Geometry check sheet. Reference: the model listing, model coordinates, mm. A direction names the side the tool comes from. Give positions to 0.01 mm unless a question says otherwise; leave off trailing zeros. Write each loop counter-clockwise with the first axis right and the second up, starting at its lowest first coordinate (ties: lowest second). Pieces come first, ordered by that corner, then holes. Notation, with made-up numbers: M 50.25,1.25 L 106.25,1.25 A26 ccw 106.25,39.25 Z; hole C 65.25,5 d8. An arc over 180 degrees is marked long. One line per item, written item: value. Start each with the question number.
1. Cross-section at B-B on y = 54. Record the cut outline in (x, z).
2. Gauge pin test, flat ends, axial feed: pin 1 (0.8 mm diameter, centred on x = -23.5, z = 4.5, fed in from -Y); pin 2 (0.9 mm diameter, centred on y = 27, z = 19.5, fed in from -X); pin 3 (0.8 mm diameter, centred on y = 25.5, z = 3.5, fed in from +X); pin 4 (2 mm diameter, centred on x = -21.5, z = 1.5, fed in from -Y). Record the tip position at first contact, or that the pin passes through.
3. Cross-section at C-C on x = -17. Count the separate pieces of the cut face and the enclosed holes in it, then the cut area to 3 significant figures.
4. Tool access check on faces 1 (the face through (-23.5, 25, 8)), 2 (the face through (-14.949, 40.313, 16.68)), 3 (the face through (-27, 12, 3)). Record the directions out of +Z, -Z, +X, -X, +Y, -Y that give a thin tool (end or side, any length) a straight path to the whole face; none if there is none.
5. Release check for a two-part mould opening along Z. For faces 4 (the face through (0, 20, -35)), 5 (the face through (18, 37, 0)), 6 (the face through (-23.49, 27.15, 10.09)), 7 (the face through (0, 40, 20)) record: pulls with the +Z half, pulls with the -Z half, needs draft (parallel to the pull), parting line crosses it, or undercut.
6. Cross-section at A-A on y = 34. Record the cut outline in (x, z), then the cut area to 3 significant figures.
7. Scan lines: line 1 (Y direction, x = 3, z = 0); line 2 (X direction, y = 46, z = 20); line 3 (Y direction, x = 12, z = -18). Record each from-to range of solid material in increasing order.
Autodesk Inventor part; units mm, degrees
ref_plane "Work Plane1" through (0, 10, 0) normal (0, -1, 0) x (1, 0, 0)
ref_plane "Work Plane3" through (0, 0, 30) normal (1, 0, 0) x (0, 0, -1)
ref_plane "Work Plane4" through (-24, 20.5, 15) normal (0, -1, 0) x (1, 0, 0)
sketch "Sketch1" plane through (0, 0, 0) normal (0, 1, 0) x (-1, 0, 0)
  line L0 (-20, 35) -> (20, 35)
  line L1 (20, 35) -> (20, -35)
  line L2 (20, -35) -> (-20, -35)
  line L3 (-20, -35) -> (-20, 35)
  line L4 (-20, 35) -> (20, -35) construction
  line L5 (20, 35) -> (-20, -35) construction
  line L6 (-17.5, 35) -> (17.5, 35)
  line L7 (17.5, 35) -> (17.5, -35)
  line L8 (17.5, -35) -> (-17.5, -35)
  line L9 (-17.5, -35) -> (-17.5, 35)
  line L10 (-17.5, 35) -> (17.5, -35) construction
  line L11 (17.5, 35) -> (-17.5, -35) construction
  line L12 (-20, 20) -> (20, 20)
  line L13 (20, 20) -> (20, -20)
  line L14 (20, -20) -> (-20, -20)
  line L15 (-20, -20) -> (-20, 20)
  line L16 (-20, 20) -> (20, -20) construction
  line L17 (20, 20) -> (-20, -20) construction
  point P0 (0, 0)
  dimension "d0" = 40
  dimension "d1" = 70
  dimension "d2" = 40
  dimension "d3" = 35
extrude "Extrusion1" add sketch "Sketch1" along normal blind 40
chamfer "Chamfer1" distance 5 angle 45 4 edges at (20, 20, 35) (-20, 20, 35) (-20, 20, -35) (20, 20, -35)
ref_plane "Work Plane1" through (0, 10, 0) normal (0, -1, 0) x (1, 0, 0)
chamfer "Chamfer2" distance 5 angle 45 2 edges at (20, 40, 0) (-20, 40, 0)
ref_plane "Work Plane3" through (0, 0, 30) normal (1, 0, 0) x (0, 0, -1)
sketch "Sketch5" plane through (0, 0, 30) normal (1, 0, 0) x (0, 0, -1)
  point P0 (30, 0)
sketch "Sketch6" plane through (0, 10, 0) normal (0, -1, 0) x (1, 0, 0)
  point P0 (0, 0)
sketch "Sketch7" plane through (0, 0, 30) normal (1, 0, 0) x (0, 0, -1)
  line L0 (-5, 40) -> (65, 40)
  line L1 (10, 40) -> (10, 60)
  line L2 (-5, 0) -> (-5, 40)
  line L3 (-5, 40) -> (-10, 45)
  line L4 (-10, 45) -> (-10, 47)
  line L5 (-10, 47) -> (-5, 52)
  line L6 (-5, 52) -> (-5, 55)
  line L7 (-5, 55) -> (-15, 55)
  line L8 (-5, 57) -> (-5, 60)
  line L9 (-5, 60) -> (10, 60)
  line L10 (-15, 57) -> (-5, 57)
  line L11 (-15, 55) -> (-15, 57)
  point P0 (30, 0)
  point P1 (-10, 46)
  point P2 (-22, 56)
  point P3 (-5, 58.5)
  point P4 (-5, 53.5)
  point P5 (-15, 56)
  point P6 (-10, 57)
  dimension "d34" = 20
  dimension "d35" = 15
  dimension "d37" = 12
  dimension "d39" = 5
  dimension "d40" = 2
  dimension "d42" = 40
  dimension "d43" = 64
  dimension "d44" = 30
  dimension "d45" = 30
  dimension "d46" = 50
  dimension "d47" = 2
  dimension "d48" = 3
revolve "Revolution2" add sketch "Sketch7" angle 360 about axis through (0, 40, 20) along (0, 1, 0)
sketch "Sketch8" plane through (0, 60, 20) normal (0, 1, 0) x (1, 0, 0)
  point P0 (0, 20)
  point P1 (0, 0)
hole "Hole1" at (0, 60, 20) direction (0, -1, 0) diameter 27 depth 20
sketch "Sketch9" plane through (-20, 0, -30) normal (-1, 0, 0) x (0, 0, 1)
  circle A0 centre (50, 27.008) radius 2.4494
  point P0 (30, 0)
extrude "Extrusion4" add sketch "Sketch9" along normal blind 5
fillet "Fillet1" radius 1 1 edges at (-25, 27.008, 17.5506)
sketch "Sketch10" plane through (-20, 0, -30) normal (-1, 0, 0) x (0, 0, 1)
  line L0 (33, 29) -> (45, 29)
  line L1 (45, 29) -> (45, 19)
  line L2 (45, 19) -> (33, 19)
  line L3 (33, 19) -> (33, 29)
  line L4 (33, 26) -> (37, 26)
  line L5 (39, 24) -> (39, 19)
  line L6 (60, 35) -> (60, 0)
  line L7 (0, 35) -> (60, 35)
  line L8 (37, 26) -> (39, 24)
  line L9 (38.2426, 29) -> (45, 22.2426)
  line L10 (42, 30.25) -> (42, 15.4606)
  line L11 (38, 22) -> (48.4916, 22)
  line L12 (44, 22) -> (44, 19)
  point P0 (30, 0)
  point P1 (39, 26)
  point P2 (39, 21.5)
  point P3 (39, 29)
  point P4 (45, 24)
  point P5 (38, 25)
  point P6 (45, 22)
  point P7 (42, 22)
  point P8 (42, 25.2426)
  dimension "d60" = 6
  dimension "d61" = 10
  dimension "d62" = 12
  dimension "d63" = 15
  dimension "d64" = 16
  dimension "d65" = 3
  dimension "d66" = 2
  dimension "d67" = 2
  dimension "d68" = 3
  dimension "d69" = 3
  dimension "d70" = 3
  dimension "d73" = 1
extrude "Extrusion5" add sketch "Sketch10" along normal blind 4 contours L0 L9 L10 L11 L5 L8 L4 L3 | L11 L12 L2 L10 | L10 L2 L5 L11 | L1 L2 L12 L11
extrude "Extrusion6" cut sketch "Sketch10" along normal blind 3 contours L0 L9 L10 L11 L5 L8 L4 L3 | L11 L12 L2 L10 | L10 L2 L5 L11
sketch "Sketch11" plane through (-24, 0, -30) normal (-1, 0, 0) x (0, 0, 1)
  line L0 (33, 29) -> (33, 26)
  line L1 (38.2426, 29) -> (33, 29)
  line L2 (34, 26) -> (34, 29)
  line L3 (33, 29) -> (33, 26)
  line L4 (33, 26) -> (33, 25)
  line L5 (33, 25) -> (34, 25)
  line L6 (34, 25) -> (34, 26)
  line L7 (33, 30) -> (34, 30)
  line L8 (33, 29) -> (33, 30)
  line L9 (34, 30) -> (34, 29)
  point P0 (30, 0)
  point P1 (33.5, 25)
  dimension "d76" = 1
extrude "Extrusion7" add sketch "Sketch11" along normal blind 8
sketch "Sketch12" plane through (-24, 25, 4) normal (0, 0, 1) x (1, 0, 0)
  line L0 (-8.9741, 1.75) -> (-1, 1.75)
  line L1 (-1, 1.75) -> (-1, 3.25)
  line L2 (-1, 3.25) -> (-8.9741, 3.25)
  line L3 (-8.9741, 3.25) -> (-8.9741, 1.75)
  line L4 (0, 0) -> (-8, 0)
  line L5 (-8, 0) -> (-8, 5)
  point P0 (24, -25)
  point P1 (-8, 3.25)
  point P2 (-8, 1.75)
  dimension "d80" = 1.5
  dimension "d81" = 1.75
  dimension "d82" = 7
extrude "Extrusion8" cut sketch "Sketch12" against normal blind 8 contours L5 L2 L1 L0
fillet "Fillet2" radius 0.5 6 edges at (-32, 25, 3.5) (-32, 30, 3.5) (-32, 26.75, 3.5) (-32, 28.25, 3.5) (-25, 28.25, 3.5) (-25, 26.75, 3.5)
sketch "Sketch13" plane through (-20, 0, -30) normal (-1, 0, 0) x (0, 0, 1)
  point P0 (30, 0)
sketch "Sketch14" plane through (-20, 0, -30) normal (-1, 0, 0) x (0, 0, 1)
  line L0 (0, 35) -> (0, 0)
  line L1 (60, 0) -> (60, 35)
  point P0 (30, 0)
sketch "Sketch15" plane through (-24, 0, -30) normal (-1, 0, 0) x (0, 0, 1)
  point P0 (30, 0)
ref_plane "Work Plane4" through (-24, 20.5, 15) normal (0, -1, 0) x (1, 0, 0)
mirror "Mirror2" about plane through (-24, 20.5, 15) normal (0, -1, 0) of "Extrusion5", "Extrusion6", "Extrusion7", "Extrusion8"
properties material "ABS Plastic"
Report:
1. outline: C 0,20 d30; hole C 0,20 d27
2. pin 1: stops at y = 12
2. pin 2: stops at x = -25
2. pin 3: stops at x = 20
2. pin 4: passes through
3. separate pieces: 3
3. enclosed holes: 0
3. area: 2,710 mm^2
4. face 1: -Z, -X
4. face 2: none
4. face 3: -Z, -X, +Y, -Y
5. face 4: pulls with the -Z half
5. face 5: needs draft
5. face 6: undercut
5. face 7: undercut
6. outline: M -20,-30 L -15,-35 L 15,-35 L 20,-30 L 20,30 L 15,35 L -15,35 L -20,30 Z
6. area: 2,750 mm^2
7. line 1: y = 0 to 40, 55 to 57
7. line 2: x = -20 to -13.5, 13.5 to 20
7. line 3: y = 0 to 40
